For this review, take the finished solid that the model builds, in its own axes (mm). Face numbers are marked on the shaded views. A direction names the side the tool comes from. Coordinates: 2 decimals unless noted, no trailing zeros. Order: outer loops, then holes, each group sorted by start corner. A loop starts at its lowest first (then second) coordinate and runs counter-clockwise, first axis right, second up.
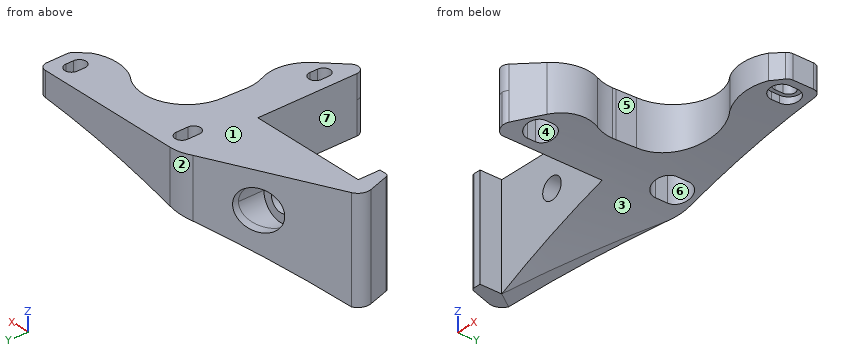
from build123d import *
from build123d.topology import SkipClean

# Parameters (mm, degrees)
RESSALTO_EXTRUS_O1_DEPTH = 6
RESSALTO_EXTRUS_O2_DEPTH = 47.171573
CORTE_EXTRUS_O1_START    = -36
CORTE_EXTRUS_O1_DEPTH    = 36
CORTE_EXTRUS_O2_START    = -6
CORTE_EXTRUS_O2_DEPTH    = 6
CORTE_EXTRUS_O3_DEPTH    = 64.000000167
ESBO_O6_R                = 2.75
CORTE_EXTRUS_O4_DEPTH    = 54.872946739
ESBO_O7_R                = 5
CORTE_EXTRUS_O5_DEPTH    = 16
RESSALTO_EXTRUS_O3_DEPTH = 56
CORTE_EXTRUS_O6_DEPTH    = 56
ESBO_O10_W               = 30
ESBO_O10_H               = 4.954017116
CORTE_EXTRUS_O7_DEPTH    = 56
ESBO_O11_W               = 2.729993951
ESBO_O11_H               = 30
CORTE_EXTRUS_O8_DEPTH    = 56
ESBO_O12_W               = 4.187219241
ESBO_O12_H               = 30
CORTE_EXTRUS_O9_DEPTH    = 56
ESBO_O13_R               = 7.968110823
CORTE_EXTRUS_O10_DEPTH   = 56
FILETE1_R                = 3
FILETE2_R                = 1
ESBO_O14_R               = 5
CORTE_EXTRUS_O11_DEPTH   = 56
CORTE_EXTRUS_O12_DEPTH   = 65.838260479


with BuildPart() as part:
    # Esboço1 → Ressalto-extrusão1 (new body)
    with BuildSketch(Plane.XY):
        with BuildLine():
            Line((-30, 24), (-2.375117905, 40.574929257))
            ThreePointArc((-2.375117905, 40.574929257), (0.100503831, 41.637149282), (2.769839649, 42))
            Line((2.769839649, 42), (40, 42))
            ThreePointArc((40, 42), (41.414213562, 41.414213562), (42, 40))
            Line((42, 40), (42, 34.828427125))
            ThreePointArc((42, 34.828427125), (41.847759065, 34.06306026), (41.414213562, 33.414213562))
            Line((41.414213562, 33.414213562), (36.670641482, 28.670641482))
            ThreePointArc((36.670641482, 28.670641482), (31.432958847, 25.911210894), (25.552715472, 26.597151419))
            ThreePointArc((25.552715472, 26.597151419), (13.045048712, 24.264475098), (10.712372391, 11.756808337))
            ThreePointArc((10.712372391, 11.756808337), (11.398312916, 5.876564962), (8.638882328, 0.638882328))
            Line((8.638882328, 0.638882328), (8, 0))
            Line((8, 0), (6.2, -1.8))
            Line((6.2, -1.8), (3.414213562, -4.585786438))
            ThreePointArc((3.414213562, -4.585786438), (1.234633135, -5.01933194), (0, -3.171572875))
            Line((0, -3.171572875), (0, 0))
            Line((0, 0), (0, 22))
            Line((0, 22), (-30, 22))
            Line((-30, 22), (-30, 24))
        make_face()
        with BuildLine():
            Line((6.2, 37.5), (6.2, 34.5))
            ThreePointArc((6.2, 34.5), (4.5, 32.8), (2.8, 34.5))
            Line((2.8, 34.5), (2.8, 37.5))
            ThreePointArc((2.8, 37.5), (4.5, 39.2), (6.2, 37.5))
        make_face(mode=Mode.SUBTRACT)
        with BuildLine():
            Line((39.2, 37.5), (39.2, 35.5))
            ThreePointArc((39.2, 35.5), (37.5, 33.8), (35.8, 35.5))
            Line((35.8, 35.5), (35.8, 37.5))
            ThreePointArc((35.8, 37.5), (37.5, 39.2), (39.2, 37.5))
        make_face(mode=Mode.SUBTRACT)
        with BuildLine():
            Line((6.2, 3.5), (6.2, 1.5))
            ThreePointArc((6.2, 1.5), (4.5, -0.2), (2.8, 1.5))
            Line((2.8, 1.5), (2.8, 3.5))
            ThreePointArc((2.8, 3.5), (4.5, 5.2), (6.2, 3.5))
        make_face(mode=Mode.SUBTRACT)
    extrude(amount=RESSALTO_EXTRUS_O1_DEPTH)

    # Esboço2 → Ressalto-extrusão2 (add, through all)
    with BuildSketch(Plane(origin=(0, 42, 0), x_dir=(1, 0, 0), z_dir=(0, 1, 0))):
        with BuildLine():
            Line((-30, 0), (-30, 20))
            ThreePointArc((-30, 20), (5.092783278, 6.734019802), (42, 0))
            Line((42, 0), (-30, 0))
        make_face()
    extrude(amount=-RESSALTO_EXTRUS_O2_DEPTH)

    # Esboço3 → Corte-extrusão1 (cut)
    with BuildSketch(Plane.XY.offset(CORTE_EXTRUS_O1_START)):
        with BuildLine():
            ThreePointArc((2.8, 34.5), (4.5, 32.8), (6.2, 34.5))
            Line((6.2, 34.5), (6.2, 37.5))
            ThreePointArc((6.2, 37.5), (4.5, 39.2), (2.8, 37.5))
            Line((2.8, 37.5), (2.8, 34.5))
        make_face()
        with BuildLine():
            Line((0, -3.171572875), (0, 22))
            Line((0, 22), (-30, 22))
            Line((-30, 22), (-30, -5.171572875))
            Line((-30, -5.171572875), (2, -5.171572875))
            ThreePointArc((2, -5.171572875), (0.585786438, -4.585786438), (0, -3.171572875))
        make_face()
        with BuildLine():
            ThreePointArc((3.414213562, -4.585786438), (2.765366865, -5.01933194), (2, -5.171572875))
            Line((2, -5.171572875), (42, -5.171572875))
            Line((42, -5.171572875), (42, 34.828427125))
            ThreePointArc((42, 34.828427125), (41.847759065, 34.06306026), (41.414213562, 33.414213562))
            Line((41.414213562, 33.414213562), (36.670641482, 28.670641482))
            ThreePointArc((36.670641482, 28.670641482), (31.432958847, 25.911210894), (25.552715472, 26.597151419))
            ThreePointArc((25.552715472, 26.597151419), (13.045048712, 24.264475098), (10.712372391, 11.756808337))
            ThreePointArc((10.712372391, 11.756808337), (11.398312916, 5.876564962), (8.638882328, 0.638882328))
            Line((8.638882328, 0.638882328), (3.414213562, -4.585786438))
        make_face()
        with BuildLine():
            ThreePointArc((35.8, 35.5), (37.5, 33.8), (39.2, 35.5))
            Line((39.2, 35.5), (39.2, 37.5))
            ThreePointArc((39.2, 37.5), (37.5, 39.2), (35.8, 37.5))
            Line((35.8, 37.5), (35.8, 35.5))
        make_face()
        with BuildLine():
            ThreePointArc((2.8, 1.5), (4.5, -0.2), (6.2, 1.5))
            Line((6.2, 1.5), (6.2, 3.5))
            ThreePointArc((6.2, 3.5), (4.5, 5.2), (2.8, 3.5))
            Line((2.8, 3.5), (2.8, 1.5))
        make_face()
        with BuildLine():
            Line((-30, 42), (-30, 24))
            Line((-30, 24), (-2.375117905, 40.574929257))
            ThreePointArc((-2.375117905, 40.574929257), (0.100503831, 41.637149282), (2.769839649, 42))
            Line((2.769839649, 42), (-30, 42))
        make_face()
    extrude(amount=CORTE_EXTRUS_O1_DEPTH, mode=Mode.SUBTRACT)

    # Esboço4 → Corte-extrusão2 (cut)
    with BuildSketch(Plane.XY.offset(CORTE_EXTRUS_O2_START)):
        with BuildLine():
            Line((42, 40), (42, 42))
            Line((42, 42), (40, 42))
            ThreePointArc((40, 42), (41.414213562, 41.414213562), (42, 40))
        make_face()
    extrude(amount=CORTE_EXTRUS_O2_DEPTH, mode=Mode.SUBTRACT)

    # Esboço5 → Corte-extrusão3 (cut, through all)
    with BuildSketch(Plane.XY.offset(1)):
        with BuildLine():
            Line((1.3, 37.5), (1.3, 34.5))
            ThreePointArc((1.3, 34.5), (4.5, 31.3), (7.7, 34.5))
            Line((7.7, 34.5), (7.7, 37.5))
            ThreePointArc((7.7, 37.5), (4.5, 40.7), (1.3, 37.5))
        make_face()
        with BuildLine():
            Line((40.2, 35.5), (40.2, 37.5))
            ThreePointArc((40.2, 37.5), (37.5, 40.2), (34.8, 37.5))
            Line((34.8, 37.5), (34.8, 35.5))
            ThreePointArc((34.8, 35.5), (37.5, 32.8), (40.2, 35.5))
        make_face()
        with BuildLine():
            Line((1.8, 3.5), (1.8, 1.5))
            ThreePointArc((1.8, 1.5), (4.5, -1.2), (7.2, 1.5))
            Line((7.2, 1.5), (7.2, 3.5))
            ThreePointArc((7.2, 3.5), (4.5, 6.2), (1.8, 3.5))
        make_face()
    extrude(amount=-CORTE_EXTRUS_O3_DEPTH, mode=Mode.SUBTRACT)

    # Esboço6 → Corte-extrusão4 (cut, through all)
    with BuildSketch(Plane.XZ.offset(-22)):
        with Locations((-15, -3)):
            Circle(ESBO_O6_R)
    extrude(amount=-CORTE_EXTRUS_O4_DEPTH, mode=Mode.SUBTRACT)

    # Esboço7 → Corte-extrusão5 (cut)
    with BuildSketch(Plane(origin=(0, 29, 0), x_dir=(-1, 0, 0), z_dir=(0, -1, 0))):
        with Locations(Location((15, 3, 0), (0, 0, 180))):
            Circle(ESBO_O7_R)
    extrude(amount=-CORTE_EXTRUS_O5_DEPTH, mode=Mode.SUBTRACT)

    # Esboço8 → Ressalto-extrusão3 (add)
    with BuildSketch(Plane.XY.offset(6)):
        Polygon((-30, 22), (-30, 16.475897374), (-32.468121282, 16.475897374), (-35.151943697, 24.974668355), (-2.375117905, 40.574929257), align=None)
    extrude(amount=-RESSALTO_EXTRUS_O3_DEPTH)

    # Esboço9 → Corte-extrusão6 (cut)
    with BuildSketch(Plane(origin=(-19.527562648, 29.041651157, 0), x_dir=(0.8298484461977135, 0.5579888496585221, 0), z_dir=(0.5579888496585221, -0.8298484461977135, 0))):
        with BuildLine():
            Line((20.669370198, -50), (20.669370198, -8.960218673))
            add(Edge.make_bspline(
                [(20.669370198, -8.960218673), (3.547051305, -13.487974371), (-12.619698693, -20)],
                knots=[1.879279318, 1.879279318, 1.879279318, 2.02269118, 2.02269118, 2.02269118], degree=2, weights=[1, 0.997430231, 1]))
            Line((-12.619698693, -20), (-12.619698693, -50))
            Line((-12.619698693, -50), (20.669370198, -50))
        make_face()
    extrude(amount=-CORTE_EXTRUS_O6_DEPTH, mode=Mode.SUBTRACT)

    # Esboço10 → Corte-extrusão7 (cut)
    with BuildSketch(Plane(origin=(-10.472437352, -7.041651157, 0), x_dir=(0, 0, -1), z_dir=(0.8298484461977135, 0.5579888496585221, 1.5073885260129385e-15))):
        with Locations((35, 37.473339864)):
            Rectangle(ESBO_O10_W, ESBO_O10_H)
    extrude(amount=-CORTE_EXTRUS_O7_DEPTH, mode=Mode.SUBTRACT)

    # Esboço11 → Corte-extrusão8 (cut)
    with BuildSketch(Plane(origin=(-22.291848959, 33.152734563, 0), x_dir=(0.8298484461977135, 0.5579888496585221, 0), z_dir=(0.5579888496585221, -0.8298484461977135, 0))):
        with Locations((-13.984695669, -35)):
            Rectangle(ESBO_O11_W, ESBO_O11_H)
    extrude(amount=-CORTE_EXTRUS_O8_DEPTH, mode=Mode.SUBTRACT)

    # Esboço12 → Corte-extrusão9 (cut)
    with BuildSketch(Plane(origin=(-19.527562648, 29.041651157, 0), x_dir=(0.8298484461977135, 0.5579888496585221, 0), z_dir=(-0.5579888496585221, 0.8298484461977135, 0))):
        with Locations((-14.713308314, 35)):
            Rectangle(ESBO_O12_W, ESBO_O12_H)
    extrude(amount=-CORTE_EXTRUS_O9_DEPTH, mode=Mode.SUBTRACT)

    # Esboço13 → Corte-extrusão10 (cut)
    with BuildSketch(Plane(origin=(0, 0, -20), x_dir=(-1, 0, 0), z_dir=(0, 0, -1))):
        with Locations((34.361612589, 20.650995678)):
            Circle(ESBO_O13_R)
    extrude(amount=CORTE_EXTRUS_O10_DEPTH, mode=Mode.SUBTRACT)

    # Filete1
    filete1_edges = [part.edges().sort_by_distance(p)[0] for p in [
        (-35.151943697, 24.974668355, -7),
    ]]
    fillet(filete1_edges, radius=FILETE1_R)

    # Filete2
    filete2_edges = [part.edges().sort_by_distance(p)[0] for p in [
        (-32.468121282, 16.475897374, -7),
    ]]
    fillet(filete2_edges, radius=FILETE2_R)

    # Esboço14 → Corte-extrusão11 (cut)
    with SkipClean():  # the faces are left unmerged after this step: merging them gives an invalid solid
        with BuildSketch(Plane(origin=(0, 29, 0), x_dir=(1, 0, 0), z_dir=(0, 1, 0))):
            with Locations((-15, 3)):
                Circle(ESBO_O14_R)
        extrude(amount=CORTE_EXTRUS_O11_DEPTH, mode=Mode.SUBTRACT)

    # Esboço15 → Corte-extrusão12 (cut, through all)
    with SkipClean():  # the faces are left unmerged after this step: merging them gives an invalid solid
        with BuildSketch(Plane.XY.offset(6)):
            with BuildLine():
                Line((9.75, 16.30952381), (10, 22.2))
                ThreePointArc((10, 22.2), (16.149553965, 32.072850311), (27.722395139, 30.906859571))
                ThreePointArc((27.722395139, 30.906859571), (33.400143909, 29.493959096), (39.042427522, 31.042427522))
                Line((39.042427522, 31.042427522), (40.056737405, 6.935592927))
                Line((40.056737405, 6.935592927), (14.498143353, 9.675700977))
                Line((14.498143353, 9.675700977), (9.75, 16.30952381))
            make_face()
        extrude(amount=-CORTE_EXTRUS_O12_DEPTH, mode=Mode.SUBTRACT)


solid = part.part
1. Clearance check with flat-ended pins moving along their axes: pin 1 Ø6 at (x, y) = (36.5, 37.5) entering from -Z; pin 2 Ø2 at (y, z) = (3, -4.5) entering from +X; pin 3 Ø1.6 at (y, z) = (2, 3.5) entering from -X. State where each tip first meets the part, or that it passes through.
Answer below:
pin 1: stops at z = -0.94
pin 2: stops at x = 10.85
pin 3: stops at x = 0
2. Take a section at D-D, the plane y = -2. Give the boundary of the cut face in (x, z), plus the area to 3 significant figures.
Answer below:
outline: (0, -8.22) arc R207.62 cw to (6, -6.48) - (6, 6) - (0, 6) - close
area: 80.0 mm2
3. Take a section at C-C, the plane z = 3.75. Give the number of separate pieces and of enclosed holes in the cut face, plus the area to 3 significant figures.
Answer below:
separate pieces: 1
enclosed holes: 3
area: 1,170 mm2
4. To check wall thickness, follow L1, parallel to X at y = 32, z = -3.25; L2, parallel to Z at x = -15, y = 30.5; L3, parallel to X at y = 1.5, z = -3.25. State the ranges of each line that lie inside material, in increasing order.
Answer below:
L1: x = -20.39 to -19.99, -10.01 to 2.5, 6.5 to 16
L2: z = -13.44 to -8, 2 to 6
L3: x = 0 to 1.8, 7.2 to 9.41
5. Take a section at A-A, the plane y = 19.5. Give the boundary of the cut face in (x, z), plus the area to 3 significant figures.
Answer below:
outline: (-33.42, -20) - (-30, -20) - (-30, 6) - (-33.42, 6) - close; (0, -8.22) arc R207.62 cw to (9.89, -5.46) - (9.89, 6) - (0, 6) - close
area: 216 mm2
6. Machinability: for the marked faces 5, 6 and 7, which of the approach directions +Z, -Z, +X, -X, +Y, -Y give a long, thin tool a straight path to every point of the face, cutting with its end or side? Answer none if there is none.
Answer below:
face 5: +Z, -Z, +X
face 6: -Z
face 7: +Z, -Z, -Y
7. The part is to be moulded in two halves that separate along X. For the marked faces 1, 2, 3 and 4, say which applies: +X half, -X half, draft (parallel to the pull), parting line (faces both ways), or undercut.
Answer below:
face 1: draft
face 2: -X half
face 3: +X half
face 4: undercut
8. Take a section at B-B, the plane x = 37.5. Give the boundary of the cut face in (y, z), plus the area to 3 significant figures.
Answer below:
outline: (30.3, -0.46) - (32.8, -0.46) - (32.8, 1) - (33.8, 1) - (33.8, 6) - (30.3, 6) - close; (39.2, 1) - (40.2, 1) - (40.2, -0.46) - (42, -0.46) - (42, 6) - (39.2, 6) - close
area: 37.8 mm2
